```python
from build123d import *

# Parameters (mm, degrees)
CROQUIS1_W              = 20
CROQUIS1_H              = 27.748412894
CROQUIS1_R              = 7.5
SALIENTE_EXTRUIR1_DEPTH = 50
CORTAR_EXTRUIR4_DEPTH   = 50
CORTAR_EXTRUIR6_DEPTH   = 12.5
CHAFL_N3_START          = -1
CHAFL_N3_OUTLINE_W      = 79
CHAFL_N3_OUTLINE_H      = 9
CHAFL_N3_DEPTH          = 2.185479897
CHAFL_N4_SIZE           = 2
CHAFL_N4_SIZE_2         = 2.02158655
CHAFL_N5_START          = -33
CHAFL_N5_OUTLINE_W      = 90
CHAFL_N5_OUTLINE_H      = 7
CHAFL_N5_DEPTH          = 2.187491538
CHAFL_N6_START          = -47
CHAFL_N6_OUTLINE_W      = 78
CHAFL_N6_OUTLINE_H      = 9
CHAFL_N6_DEPTH          = 1.956109558
CHAFL_N9_START          = -12
CHAFL_N9_OUTLINE_W      = 79
CHAFL_N9_OUTLINE_H      = 9
CHAFL_N9_DEPTH          = 2.225324788
CHAFL_N10_START         = -36
CHAFL_N10_OUTLINE_W     = 65
CHAFL_N10_OUTLINE_H     = 9
CHAFL_N10_DEPTH         = 1.916264666
CROQUIS17_W             = 6
CROQUIS17_H             = 25
CORTAR_EXTRUIR8_DEPTH   = 50
CORTAR_EXTRUIR9_DEPTH   = 12.5
CORTAR_EXTRUIR10_DEPTH  = 12.5
CROQUIS22_W             = 25
CROQUIS22_H             = 11.323267037
CORTAR_EXTRUIR11_DEPTH  = 128.16446319
CROQUIS23_W             = 25
CROQUIS23_H             = 16.343664216
CORTAR_EXTRUIR12_DEPTH  = 80
CHAFL_N17_SIZE          = 9
CHAFL_N17_SIZE_2        = 8.307561118


with BuildPart() as part:
    # Croquis1 → Saliente-Extruir1 (new body)
    # profile 1 of 4: a face of its own
    with BuildSketch(Plane.XY):
        with BuildLine():
            Line((-57.030721287, -14.034703102), (-41.84315615, 0))
            Line((-41.84315615, 0), (-41.84315615, -15.5))
            Line((-41.84315615, -15.5), (-56.84315615, -15.5))
            add(Edge.make_bspline(
                [(-57.030721287, -14.034703102), (-57.299191115, -14.282793846), (-57.220648616, -14.896383781), (-57.142106118, -15.509973716), (-56.84315615, -15.5)],
                knots=[0.390549282, 0.390549282, 0.390549282, 1.766070968, 1.766070968, 3.141592654, 3.141592654, 3.141592654], degree=2, weights=[1, 0.772669387, 1, 0.772669387, 1]))
        make_face()
    # profile 2 of 4: a face of its own
    with BuildSketch(Plane.XY):
        Polygon((28.15684385, -21.624206447), (28.15684385, 6.124206447), (-41.84315615, 0), (-41.84315615, -15.5), align=None)
    # profile 3 of 4: a face of its own
    with BuildSketch(Plane.XY):
        with Locations((38.15684385, -7.75)):
            Rectangle(CROQUIS1_W, CROQUIS1_H)
    # profile 4 of 4: a face of its own
    with BuildSketch(Plane.XY):
        with BuildLine():
            Line((48.15684385, -21.624206447), (83.15684385, -21.624206447))
            ThreePointArc((83.15684385, -21.624206447), (97.031050296, -7.75), (83.15684385, 6.124206447))
            Line((83.15684385, 6.124206447), (48.15684385, 6.124206447))
            Line((48.15684385, 6.124206447), (48.15684385, -21.624206447))
        make_face()
        with Locations((83.15684385, -7.75)):
            Circle(CROQUIS1_R, mode=Mode.SUBTRACT)
    extrude(amount=SALIENTE_EXTRUIR1_DEPTH)

    # Croquis6 → Cortar-Extruir4 (cut)
    with BuildSketch(Plane(origin=(0, 6.124206447, 0), x_dir=(1, 0, 0), z_dir=(0, 1, 0))):
        Polygon((83.15684385, 0), (28.15684385, 0), (28.15684385, -3.845974657), align=None)
        Polygon((83.15684385, -50), (28.15684385, -46.154025343), (28.15684385, -50), align=None)
        Polygon((28.15684385, -50), (28.15684385, -46.154025343), (-41.84315615, -37.55910608), (-41.84315615, -50), align=None)
        Polygon((28.15684385, -3.845974657), (28.15684385, 0), (-41.84315615, 0), (-41.84315615, -12.44089392), align=None)
        Polygon((-57.233399119, 0), (-41.84315615, 0), (-41.84315615, -12.44089392), (-57.030721287, -17.968715561), (-57.233399119, -17.968715561), align=None)
        Polygon((-57.233399119, -32.031284439), (-57.233399119, -50), (-41.84315615, -50), (-41.84315615, -37.55910608), (-57.030721287, -32.031284439), align=None)
    extrude(amount=-CORTAR_EXTRUIR4_DEPTH, mode=Mode.SUBTRACT)

    # Croquis10 → Cortar-Extruir6 (cut, symmetric)
    with BuildSketch(Plane.XY.offset(25)):
        with BuildLine():
            Line((83.15684385, 6.124206447), (75.731562774, 6.124206447))
            Line((75.731562774, 6.124206447), (75.731562774, 3.970017299))
            ThreePointArc((75.731562774, 3.970017299), (69.289041207, -8.171490688), (76.457035077, -19.899327839))
            Line((76.457035077, -19.899327839), (76.457035077, -21.624206447))
            Line((76.457035077, -21.624206447), (83.15684385, -21.624206447))
            ThreePointArc((83.15684385, -21.624206447), (97.031050296, -7.75), (83.15684385, 6.124206447))
        make_face()
    extrude(amount=CORTAR_EXTRUIR6_DEPTH, both=True, mode=Mode.SUBTRACT)

    # Chaflán3: read off the stored shape, not the designer's step
    # Chaflán3 outline → Chaflán3 (cut)
    with BuildSketch(Plane(origin=(0, 0, 0), x_dir=(0.9987827677655402, 0.0349207435267313, -0.034835678350610806), z_dir=(0.04932527561612769, -0.7071067811865458, 0.7053843046066418)).offset(CHAFL_N3_START)):
        with Locations((51.5, 5.5)):
            Rectangle(CHAFL_N3_OUTLINE_W, CHAFL_N3_OUTLINE_H)
    extrude(amount=CHAFL_N3_DEPTH, mode=Mode.SUBTRACT)

    # Chaflán4
    # the kernel refuses this chamfer: 2.02158655, 2 mm, written as the material it takes off along each edge
    with BuildSketch(Plane(origin=(29.320006018, 6.22596995, 3.703156301), x_dir=(0.1209504317481252, 0.010581791626527273, 0.9926021452454729), z_dir=(-0.9888249944080325, -0.08651097722179166, 0.1214124427482008))) as chafl_n4_piece_1:
        Polygon((CHAFL_N4_SIZE, 0), (-CHAFL_N4_SIZE_2 * 0.0106216131418, -CHAFL_N4_SIZE_2 * 0.999943588993), (0, 0), align=None)
    extrude(amount=87.568441366, mode=Mode.SUBTRACT)

    # Chaflán5: read off the stored shape, not the designer's step
    # Chaflán5 outline → Chaflán5 (cut)
    with BuildSketch(Plane(origin=(0, 0, 0), x_dir=(0.9891526601001411, 0.10461310355007251, 0.1031169897855652), z_dir=(0.14689116725254298, -0.7044557654033778, -0.6943810622224129)).offset(CHAFL_N5_START)):
        with Locations((4, 27.5)):
            Rectangle(CHAFL_N5_OUTLINE_W, CHAFL_N5_OUTLINE_H)
    extrude(amount=CHAFL_N5_DEPTH, mode=Mode.SUBTRACT)

    # Chaflán6: read off the stored shape, not the designer's step
    # Chaflán6 outline → Chaflán6 (cut)
    with BuildSketch(Plane(origin=(0, 0, 0), x_dir=(0.9987827677655402, -0.034920743526731114, 0.03483567835061047), z_dir=(0.04932527561612732, 0.7071067811865474, -0.7053843046066404)).offset(CHAFL_N6_START)):
        with Locations((54, -18.5)):
            Rectangle(CHAFL_N6_OUTLINE_W, CHAFL_N6_OUTLINE_H)
    extrude(amount=CHAFL_N6_DEPTH, mode=Mode.SUBTRACT)

    # Chaflán9: read off the stored shape, not the designer's step
    # Chaflán9 outline → Chaflán9 (cut)
    with BuildSketch(Plane(origin=(0, 0, 0), x_dir=(0.9987827677655402, -0.03492074352673121, -0.03483567835061067), z_dir=(0.049325275616127526, 0.7071067811865464, 0.7053843046066414)).offset(CHAFL_N9_START)):
        with Locations((52.5, -16.5)):
            Rectangle(CHAFL_N9_OUTLINE_W, CHAFL_N9_OUTLINE_H)
    extrude(amount=CHAFL_N9_DEPTH, mode=Mode.SUBTRACT)

    # Chaflán10: read off the stored shape, not the designer's step
    # Chaflán10 outline → Chaflán10 (cut)
    with BuildSketch(Plane(origin=(0, 0, 0), x_dir=(0.9987827677655402, 0.03492074352673113, 0.034835678350610584), z_dir=(0.049325275616127415, -0.7071067811865462, -0.7053843046066413)).offset(CHAFL_N10_START)):
        with Locations((60.5, 29.5)):
            Rectangle(CHAFL_N10_OUTLINE_W, CHAFL_N10_OUTLINE_H)
    extrude(amount=CHAFL_N10_DEPTH, mode=Mode.SUBTRACT)

    # Croquis17 → Cortar-Extruir8 (cut, symmetric)
    with BuildSketch(Plane(origin=(0, 0, 0), x_dir=(1, 0, 0), z_dir=(0, 1, 0))):
        with Locations((76.444203312, -25)):
            Rectangle(CROQUIS17_W, CROQUIS17_H)
    extrude(amount=CORTAR_EXTRUIR8_DEPTH, both=True, mode=Mode.SUBTRACT)

    # Croquis19 → Cortar-Extruir9 (cut, symmetric)
    with BuildSketch(Plane.XY.offset(25)):
        Polygon((83.15684385, 6.124206447), (83.15684385, -7.75), (63.342423567, 6.124206447), align=None)
        Polygon((63.342423567, -21.624206447), (83.15684385, -7.75), (83.15684385, -21.624206447), align=None)
    extrude(amount=CORTAR_EXTRUIR9_DEPTH, both=True, mode=Mode.SUBTRACT)

    # Croquis20 → Cortar-Extruir10 (cut, symmetric)
    with BuildSketch(Plane.XY.offset(25)):
        with BuildLine():
            Line((61.272360576, 6.124206447), (69.282637403, -7.75))
            ThreePointArc((69.282637403, -7.75), (73.346298387, 2.060545462), (83.15684385, 6.124206447))
            Line((83.15684385, 6.124206447), (61.272360576, 6.124206447))
        make_face()
        with BuildLine():
            ThreePointArc((83.15684385, -21.624206447), (73.346298387, -17.560545462), (69.282637403, -7.75))
            Line((69.282637403, -7.75), (61.272360576, -21.624206447))
            Line((61.272360576, -21.624206447), (83.15684385, -21.624206447))
        make_face()
    extrude(amount=CORTAR_EXTRUIR10_DEPTH, both=True, mode=Mode.SUBTRACT)

    # Croquis22 → Cortar-Extruir11 (cut, through all)
    with BuildSketch(Plane(origin=(48.606129612, 28.062762016, 0), x_dir=(0, 0, -1), z_dir=(0.866025403784436, 0.5000000000000046, 0))):
        with Locations((-25, -47.0146491)):
            Rectangle(CROQUIS22_W, CROQUIS22_H)
    extrude(amount=-CORTAR_EXTRUIR11_DEPTH, mode=Mode.SUBTRACT)

    # Croquis23 → Cortar-Extruir12 (cut)
    with BuildSketch(Plane(origin=(100, 0, 0), x_dir=(0, 0, -1), z_dir=(1, 0, 0))):
        with Locations((-25, -20.921832108)):
            Rectangle(CROQUIS23_W, CROQUIS23_H)
    extrude(amount=-CORTAR_EXTRUIR12_DEPTH, mode=Mode.SUBTRACT)

    # Chaflán14
    # the kernel refuses this chamfer: 5 mm, written as the material it takes off along each edge
    with BuildSketch(Plane(origin=(60.622383365, -12.75, 37.5), x_dir=(0.8660254037844363, 0.5000000000000041, 0), z_dir=(0, 0, -1))) as chafl_n14_piece_1:
        with BuildLine():
            Line((1.532931127, 0.051763809), (-1.353439203, -0.72163679))
            Line((-1.353439203, -0.72163679), (-1.403439203, -0.63503425))
            ThreePointArc((-1.403439203, -0.63503425), (-0.713778649, -0.296630241), (-0.05, 0.08660254))
            Line((-0.05, 0.08660254), (0, 0.1))
            ThreePointArc((0, 0.1), (0.766465564, 0.1), (1.532931127, 0.151763809))
            Line((1.532931127, 0.151763809), (1.532931127, 0.051763809))
        make_face()
    extrude(amount=25, mode=Mode.SUBTRACT)

    # Chaflán15
    # the kernel refuses this chamfer: 5 mm, written as the material it takes off along each edge
    with BuildSketch(Plane(origin=(61.272360576, 6.124206447, 12.5), x_dir=(-1, 0, 0), z_dir=(0, 0, 1))) as chafl_n15_piece_1:
        with BuildLine():
            Line((3.059956427, -0.1), (-1.616580754, 2.6))
            Line((-1.616580754, 2.6), (-1.703183294, 2.55))
            ThreePointArc((-1.703183294, 2.55), (-0.851591647, 1.275), (-0.08660254, -0.05))
            Line((-0.08660254, -0.05), (0, -0.1))
            ThreePointArc((0, -0.1), (1.529978213, -0.1), (3.059956427, -0.2))
            Line((3.059956427, -0.2), (3.059956427, -0.1))
        make_face()
    extrude(amount=25, mode=Mode.SUBTRACT)

    # Chaflán17
    # the kernel refuses this chamfer: 9, 8.307561118 mm, written as the material it takes off along each edge
    with BuildSketch(Plane(origin=(20, -20.91057508, 12.5), x_dir=(-0.9961946980917451, 0.08715574274766211, 0), z_dir=(0, 0, 1))) as chafl_n17_piece_1_section:
        Polygon((CHAFL_N17_SIZE, 0), (CHAFL_N17_SIZE_2 * 0.0871557427526, -CHAFL_N17_SIZE_2 * 0.996194698149), (0, 0), align=None)
    chafl_n17_piece_1 = extrude(amount=25, mode=Mode.PRIVATE)
    chafl_n17_piece_1 = split(chafl_n17_piece_1, bisect_by=Plane(origin=(20, -12.75, 12.5), z_dir=(0, -1, 0)), keep=Keep.TOP, mode=Mode.PRIVATE)
    add(chafl_n17_piece_1, mode=Mode.SUBTRACT)


solid = part.part
```
Model file for the job. Use its own axes, mm. A direction names the side the tool comes from. Round coordinates to 2 decimals unless told otherwise and drop trailing zeros. Loops run counter-clockwise (first coordinate to the right, second up) from the corner with the lowest first, then second, coordinate; pieces in that order, holes last. Notation, with made-up numbers: M 78,69 L 117,69 A29 cw 117,105 Z; hole C 36.25,-28.5 d5. An arc over 180 degrees is marked long. Put each result on its own line as item: value. Start each with the question number.
Item 1: Mould opens along X. For faces 4 (the face through (60.55, -12.41, 25.18)), 5 (the face through (75.664, -7.42, 6.162)), 6 (the face through (56, -7.6, 48.1)) say: released by +X, released by -X, zero draft, split by the parting line, or undercut.
Item 2: Cut at A-A (y = -4.5). List the corners of the cut face in (x, z).
Item 3: 3-axis set-ups, long thin cutter, end or side, ignore diameter. For faces 1 (the face through (-8.17, 1.9, 40.72)), 2 (the face through (60.52, 4.89, 24.82)), 3 (the face through (40, -12.75, 25)): which of +Z, -Z, +X, -X, +Y, -Y reach the whole face in a straight line?
Item 4: Drill centre lines: line 1 along Y through (x, z) = (42, 14); line 2 along Z through (x, y) = (72, -11); line 3 along Y through (x, z) = (89, 39.5). Where is each one in solid material? Low to high.
Item 5: Cut at B-B (x = 72.5). List the corners of the cut face in (y, z), then the cut area to 3 significant figures.
Item 6: Cut at D-D (x = -12). List the corners of the cut face in (y, z), then the cut area to 3 significant figures.
Item 7: Drop flat-ended pins along their axis: P1, Ø13.5, axis at x = 83.16, y = -7.75, coming from the +Z side; P2, Ø8, axis at x = 16, y = -14.5, coming from the +Z side; P3, Ø12.5, axis at x = 37, z = 21.5, coming from the -Y side; P4, Ø10, axis at y = -18.5, z = 18.5, coming from the +X side. Give the stop position or say it passes through.
Item 8: Cut at C-C (y = -17.25). List the corners of the cut face in (x, z), then the cut area to 3 significant figures.
Answer block:
1. face 4: released by +X
1. face 5: undercut
1. face 6: released by -X
2. outline: M -46.71,14.21 L -41.84,12.44 L 28.16,3.85 L 76.4,0.47 L 76.4,12.5 L 67.41,12.5 L 67.41,37.5 L 76.4,37.5 L 76.4,49.53 L 28.16,46.15 L -41.84,37.56 L -46.71,35.79 Z; M 89.92,0 L 96.65,0 L 96.65,12.5 L 89.92,12.5 Z; M 89.92,37.5 L 96.65,37.5 L 96.65,50 L 89.92,50 Z
3. face 1: +Z, -X, +Y
3. face 2: +X, +Y
3. face 3: +X, -Y
4. line 1: -12.75 to 6.12
4. line 2: 0.78 to 12.5, 37.5 to 49.22
4. line 3: -20.33 to -12.45, -3.05 to 4.83
5. outline: M -21.62,2.75 L -19.62,0.75 L 4.12,0.75 L 6.12,2.75 L 6.12,12.5 L -21.62,12.5 Z; M -21.62,37.5 L 6.12,37.5 L 6.12,47.25 L 4.12,49.25 L -19.62,49.25 L -21.62,47.25 Z
5. area: 644 mm2
6. outline: M -18.11,8.78 L 0.58,8.78 L 2.61,10.79 L 2.61,39.19 L 0.6,41.22 L -18.11,41.22 Z
6. area: 668 mm2
7. P1: through
7. P2: z = 45.15
7. P3: y = -12.75
7. P4: x = 18.93
8. outline: M -21.84,9.98 L 28.16,3.85 L 83.16,0 L 93.27,0 L 93.27,12.5 L 14.46,12.5 L 14.46,37.5 L 93.27,37.5 L 93.27,50 L 83.16,50 L 28.16,46.15 L -21.84,40.02 Z
8. area: 2,880 mm2
